Geometry check sheet. Reference: the model listing, model coordinates, mm. Round coordinates to 2 decimals unless told otherwise and drop trailing zeros. Loops run counter-clockwise (first coordinate to the right, second up) from the corner with the lowest first, then second, coordinate; pieces in that order, holes last. Notation, with made-up numbers: (-27.75, -27.5) - (17.25, -27.5) arc R20 ccw to (17.25, -23.5) - close; hole circle Ø9 at (50.5, -27). An arc over 180 degrees is marked (long way). Answer in a Markdown table with one row per item. Add a question column.
```python
from build123d import *

# Parameters (mm, degrees)
F0_W     = 545.846
F0_H     = 273.05
F1_DEPTH = 317.5
F4_DEPTH = 545.847
F5_DEPTH = 273.051


with BuildPart() as f1:
    # F0 (on Top) → F1 (new body)
    with BuildSketch(Plane.XY):
        with Locations((18.801767, 15.887847)):
            Rectangle(F0_W, F0_H)
    extrude(amount=F1_DEPTH)

    # F3 (on face) → F4 (cut, through all)
    with BuildSketch(Plane(origin=(-254.121233, 0, 0), x_dir=(0, -1, 0), z_dir=(-1, 0, 0))):
        Polygon((-103.856937, 92.9894), (-152.412847, 92.9894), (-152.412847, 0), (120.637153, 0), (120.637153, 317.5), align=None)
    extrude(amount=-F4_DEPTH, mode=Mode.SUBTRACT)

    # F2 (on face) → F5 (cut, through all)
    with BuildSketch(Plane(origin=(0, 152.412847, 0), x_dir=(-1, 0, 0), z_dir=(0, 1, 0))):
        Polygon((-63.378767, 0), (25.775233, 0), (254.121233, 0), (254.121233, 317.5), (29.610633, 92.9894), (-67.214167, 92.9894), (-291.724767, 317.5), (-291.724767, 0), align=None)
    extrude(amount=-F5_DEPTH, mode=Mode.SUBTRACT)


solid = f1.part
```
Q1. Cross-section at B-B, the plane z = 290.5. Enter the section's corners in (x, y), plus the area to 3 significant figures.
Q2. Depth check by flat-ended pin: P1, Ø2, axis at y = 97.5, z = 273, coming from the +X side; P2, Ø1, axis at x = 56, y = -92.5, coming from the -Z side; P3, Ø2, axis at x = 172.5, y = 99, coming from the -Z side. Enter the tip coordinate at first touch or a pass-through.
Q3. Scan lines: line 1 (Z direction, x = -152.5, y = 25); line 2 (Z direction, x = -88.5, y = 134.5); line 3 (X direction, y = 50, z = 298). Record each from-to range of solid material in increasing order. Write a range as from..to.
Q4. Cross-section at A-A, the plane y = -96.5. Enter the section's corners in (x, z).
Check sheet entries:
| question | item | result |
|---|---|---|
| 1 | outline | (-227.12, -93.64) - (264.72, -93.64) - (264.72, 152.41) - (-227.12, 152.41) - close |
| 1 | area | 121,000 mm² |
| 2 | P1 | x = 248.22 |
| 2 | P2 | z = 288.86 |
| 2 | P3 | z = 197.28 |
| 3 | line 1 | 215.88..317.5 |
| 3 | line 2 | 151.88..317.5 |
| 3 | line 3 | -234.62..272.22 |
| 4 | outline | (-254.12, 317.5) - (-229.98, 293.36) - (267.59, 293.36) - (291.72, 317.5) - close |
